Could you check a few things on this model? Use its own coordinates, in mm. A direction names the side the tool comes from. Coordinates: 2 decimals unless noted, no trailing zeros. Loops run counter-clockwise (first coordinate to the right, second up) from the corner with the lowest first, then second, coordinate; pieces in that order, holes last. Notation, with made-up numbers: M -24.75,24 L -14.75,24 A12 cw -14.75,32 Z; hole C 17.25,54.25 d4. An arc over 180 degrees is marked long. Return JSON: item names as keys, results as strings. Group by question number.
from build123d import *

# Parameters (mm, degrees)
F0_W     = 38.1
F0_H     = 139.7
F0_W_2   = 25.4
F0_H_2   = 127
F1_DEPTH = 12.7
F2_DEPTH = 6.35
F3_F1_R  = 5.08
F3_F2_R  = 5.08
F3_F3_R  = 5.08
F3_F4_R  = 5.08
F3_F5_R  = 5.08


# Not quite as in the source:
# - a feature of the source that left no trace in its solid (it failed there, or was rolled back) is left out


with BuildPart() as f1:
    # F0 (on Top) → F1 (new body)
    with BuildSketch(Plane.XY):
        Rectangle(F0_W, F0_H)
        Rectangle(F0_W_2, F0_H_2, mode=Mode.SUBTRACT)
    extrude(amount=F1_DEPTH)

    # F0 (on Top) → F2 (join)
    with BuildSketch(Plane.XY):
        Rectangle(F0_W_2, F0_H_2)
    extrude(amount=F2_DEPTH)

    # F3: fillet of radius 5.08 on 6 edges, made by hand

    # F3_f1
    f3_f1_edges = [f1.edges().sort_by_distance(p)[0] for p in [
        (19.05, -69.85, 6.35),
    ]]
    fillet(f3_f1_edges, radius=F3_F1_R)

    # F3_f2
    f3_f2_edges = [f1.edges().sort_by_distance(p)[0] for p in [
        (19.05, 69.85, 6.35),
    ]]
    fillet(f3_f2_edges, radius=F3_F2_R)

    # F3_f3
    f3_f3_edges = [f1.edges().sort_by_distance(p)[0] for p in [
        (-19.05, -69.85, 6.35),
    ]]
    fillet(f3_f3_edges, radius=F3_F3_R)

    # F3_f4
    f3_f4_edges = [f1.edges().sort_by_distance(p)[0] for p in [
        (-19.05, 69.85, 6.35),
    ]]
    fillet(f3_f4_edges, radius=F3_F4_R)

    # F3_f5
    f3_f5_edges = [f1.edges().sort_by_distance(p)[0] for p in [
        (0, 69.85, 0),
    ]]
    fillet(f3_f5_edges, radius=F3_F5_R)


solid = f1.part
(1) Imagine slicing it at D-D, the plane z = 2.75. Write out the boundary of the cut face in (x, y), then the cut area to 3 significant figures.
(2) If I drill on L1, parallel to X at y = -39.5, z = 10.5; L2, parallel to Y at x = 1.5, z = 10.5; L3, parallel to Z at x = 3, y = 38, over which ranges is the centre line in solid material (lowest first)? Write a range as [from, to].
(3) Imagine slicing it at B-B, the plane z = 11. Write out the boundary of the cut face in (x, y), then the cut area to 3 significant figures.
(4) We'd pull the mould along X, two halves only. Please class faces 1 (the face through (17.522, -68.401, 8.943)), 2 (the face through (-19.05, -1, 9)), 3 (the face through (0, 63.5, 9)), 4 (the face through (0, 1, 6.35)): +X half, -X half, draft (parallel to the pull), parting line (faces both ways), or undercut.
(5) For faces 5 (the face through (12.7, -1, 9)), 6 (the face through (-0.196, -68.322, 1.449)), which set-ups out of +Z, -Z, +X, -X, +Y, -Y let a thin tool reach every point of the face, with its end or its side?
(6) Imagine slicing it at A-A, the plane x = 7. Write out the boundary of the cut face in (y, z).
(7) Will these pins go through, and if not, where does the flat tip stop? P1, Ø3, axis at x = -3.5, y = -3, coming from the +Z side; P2, Ø3, axis at x = 14, z = 3, coming from the -Y side.
(8) Imagine slicing it at C-C, the plane y = 33. Write out the boundary of the cut face in (x, z), then the cut area to 3 significant figures.
Checks:
{
 "1": {"outline": "M -18.48,-64.77 A4.51 ccw -13.97,-69.28 L 13.97,-69.28 A4.51 ccw 18.48,-64.77 L 18.48,64.77 A4.51 ccw 13.97,69.28 L -13.97,69.28 A4.51 ccw -18.48,64.77 Z", "area": "5,110 mm²"},
 "2": {"L1": "[-19.05, -12.7], [12.7, 19.05]", "L2": "[-69.85, -63.5], [63.5, 69.85]", "L3": "[0, 6.35]"},
 "3": {"outline": "M -19.05,-64.77 A5.08 ccw -13.97,-69.85 L 13.97,-69.85 A5.08 ccw 19.05,-64.77 L 19.05,64.77 A5.08 ccw 13.97,69.85 L -13.97,69.85 A5.08 ccw -19.05,64.77 Z; hole M -12.7,-63.5 L 12.7,-63.5 L 12.7,63.5 L -12.7,63.5 Z", "area": "2,070 mm²"},
 "4": {"face 1": "+X half", "face 2": "-X half", "face 3": "undercut", "face 4": "undercut"},
 "5": {"face 5": "+Z", "face 6": "-Z, +X, -X, -Y"},
 "6": {"outline": "M -69.85,5.08 A5.08 ccw -64.77,0 L 64.77,0 A5.08 ccw 69.85,5.08 L 69.85,12.7 L 63.5,12.7 L 63.5,6.35 L -63.5,6.35 L -63.5,12.7 L -69.85,12.7 Z"},
 "7": {"P1": "z = 6.35", "P2": "y = -69.82"},
 "8": {"outline": "M -19.05,5.08 A5.08 ccw -13.97,0 L 13.97,0 A5.08 ccw 19.05,5.08 L 19.05,12.7 L 12.7,12.7 L 12.7,6.35 L -12.7,6.35 L -12.7,12.7 L -19.05,12.7 Z", "area": "312 mm²"}
}
